Autodesk Inventor part; units mm, degrees
ref_plane "Plan de construction2" through (22, 0, 85) normal (1, 0, 0) x (0, 1, 0)
ref_plane "Plan de construction3" through (0, -22, 85) normal (0, 1, 0) x (-1, 0, 0)
ref_plane "XY Plane" through (0, 0, 0) normal (0, 0, 1) x (1, 0, 0)
sketch "Esquisse1" plane through (0, 0, 0) normal (1, 0, 0) x (0, 1, 0)
  line L0 (0, 0) -> (0, 594.5025)
  line L1 (22, 0) -> (22, 170)
  line L2 (19, 0) -> (19, 170)
  line L3 (22, 170) -> (19, 170)
  line L4 (22, 0) -> (19, 0)
  dimension "d0" = 38
  dimension "d3" = 3
  dimension "d58" = 170
revolve "Révolution1" add sketch "Esquisse1" angle 360 about axis through (0, 0, 0) along (0, 0, 1)
sketch "Esquisse3" plane through (0, 0, 0) normal (0, 1, 0) x (-1, 0, 0)
  line L0 (-19, 170) -> (19, 170)
  line L1 (12.5, 168) -> (-12.5, 168)
  line L2 (-12.5, 168) -> (-12.5, 126)
  line L3 (-12.5, 126) -> (12.5, 126)
  line L4 (12.5, 126) -> (12.5, 168)
  point P0 (0, 0)
  point P1 (0, 168)
  point P2 (0, 170)
  dimension "d108" = 42
  dimension "d109" = 2
  dimension "d110" = 25
extrude "Extrusion2" cut sketch "Esquisse3" along normal up to surface
ref_plane "Plan de construction2" through (22, 0, 85) normal (1, 0, 0) x (0, 1, 0)
sketch "Esquisse4" plane through (22, 0, 85) normal (1, 0, 0) x (0, 1, 0)
  line L0 (-22, 85) -> (22, 85)
  point P0 (0, -85)
  point P1 (0, 79)
  dimension "d24" = 6
hole "Perçage1" at (22, 0, 164) direction (-1, 0, 0) diameter 3.4 depth 8 counterbore diameter 6.5 counterbore depth 0.5
pattern_circular "Réseau circulaire2" count 4 over 180 about axis through (0, 0, -10) along (0, 0, -1) of "Perçage1"
chamfer "Chanfrein2" distance 1 angle 45 6 edges at (-12.5, 18.1039, 147) (-6.5466, 21.0034, 126) (6.5466, 21.0034, 126) (12.5, 18.1039, 147) (-6.5466, 21.0034, 168) (6.5466, 21.0034, 168)
ref_plane "Plan de construction3" through (0, -22, 85) normal (0, 1, 0) x (-1, 0, 0)
thread "Filetage3"
properties part number "reservoir_guide"
Verification items for the finished model (mm, model axes). A direction names the side the tool comes from. Coordinates: 2 decimals unless noted, no trailing zeros. Write each loop counter-clockwise with the first axis right and the second up, starting at its lowest first coordinate (ties: lowest second). Pieces come first, ordered by that corner, then holes. Notation, with made-up numbers: (27.25, -16) - (84.25, -16) arc R18 cw to (84.25, 17) - close; hole circle Ø10 at (34.25, 45). An arc over 180 degrees is marked (long way). One line per question, with ' | ' between items. Start each with the question number.
1. Section check B-B (x = 0). Enter the section's corners in (y, z).
2. Access from +Z, -Z, +X, -X, +Y, -Y to the whole of each face (thin tool, end or side, straight path). Record for faces 5 (the cylindrical face through (21.69, -0.98, 160.9)), 6 (the cylindrical face through (9.65, -17.74, 162.38)), 7 (the flat face through (-21.5, -1.4, 162.6)), 8 (the flat face through (-0.1, 19.4, 168)).
3. Section check C-C (z = 117). Enter the section's corners in (x, y), plus the area to 3 significant figures.
4. Draft check along X on faces 1 (the flat face through (21.5, 1.4, 162.6)), 2 (the flat face through (12.5, 16, 147)), 3 (the cylindrical face through (10, -19.27, 160.9)), 4 (the flat face through (-18, -7, 0)). Enter one of: released by +X, released by -X, zero draft, split by the parting line, or undercut.
5. Gauge pin test, flat ends, axial feed: P1, Ø0.8, axis at y = 15.5, z = 154.5, coming from the +X side; P2, Ø2, axis at y = -1, z = 163.5, coming from the +X side; P3, Ø5, axis at y = 13, z = 77.5, coming from the -X side. Record the tip position at first contact, or that the pin passes through.
6. Section check D-D (z = 164). Count the separate pieces of the cut face and the enclosed holes in it, plus the area to 3 significant figures.
7. Section check A-A (y = 0). Enter the section's corners in (x, z).
8. Material ranges on line 1 along Z through (x, y) = (20.6, 0); line 2 along X through (y, z) = (-1, 152.5); line 3 along X through (y, z) = (-2.5, 23), recorded low to high.
Computed values:
1) outline: (-22, 0) - (-19, 0) - (-19, 170) - (-22, 170) - close; (19, 0) - (22, 0) - (22, 125) - (21, 126) - (19, 126) - close; (19, 168) - (21, 168) - (22, 169) - (22, 170) - (19, 170) - close
2) face 5: +X | face 6: none | face 7: -X | face 8: +Y
3) outline: circle Ø44 at (0, 0); hole circle Ø38 at (0, 0) | area: 386 mm²
4) face 1: released by +X | face 2: undercut | face 3: undercut | face 4: zero draft
5) P1: x = 16 | P2: x = 21.5 | P3: x = -19.33
6) separate pieces: 5 | enclosed holes: 0 | area: 260 mm²
7) outline: (-22, 0) - (-19, 0) - (-19, 162.3) - (-21.5, 162.3) - (-21.5, 160.75) - (-22, 160.75) - close; (-22, 167.25) - (-21.5, 167.25) - (-21.5, 165.7) - (-19, 165.7) - (-19, 170) - (-22, 170) - close; (19, 0) - (22, 0) - (22, 160.75) - (21.5, 160.75) - (21.5, 162.3) - (19, 162.3) - close; (19, 165.7) - (21.5, 165.7) - (21.5, 167.25) - (22, 167.25) - (22, 170) - (19, 170) - close
8) line 1: 0 to 162.3, 165.7 to 170 | line 2: -21.98 to -18.97, 18.97 to 21.98 | line 3: -21.86 to -18.83, 18.83 to 21.86
